from build123d import *

# Parameters (mm, degrees)
ESQUISSE1_R        = 5.74
BOSS_EXTRU_1_DEPTH = 5.5
ESQUISSE2_R        = 11.65
BOSS_EXTRU_2_DEPTH = 8
ESQUISSE3_R        = 8.55
BOSS_EXTRU_3_DEPTH = 35.3
ESQUISSE4_R        = 3.5
BOSS_EXTRU_4_DEPTH = 7.2


with BuildPart() as part:
    # Esquisse1 → Boss.-Extru.1 (new body)
    with BuildSketch(Plane.XY):
        Circle(ESQUISSE1_R)
    extrude(amount=BOSS_EXTRU_1_DEPTH)

    # Esquisse2 → Boss.-Extru.2 (add)
    with BuildSketch(Plane(origin=(0, 0, 0), x_dir=(-1, 0, 0), z_dir=(0, 0, -1))):
        Circle(ESQUISSE2_R)
    extrude(amount=BOSS_EXTRU_2_DEPTH)

    # Esquisse3 → Boss.-Extru.3 (add)
    with BuildSketch(Plane(origin=(0, 0, -8), x_dir=(-1, 0, 0), z_dir=(0, 0, -1))):
        Circle(ESQUISSE3_R)
    extrude(amount=BOSS_EXTRU_3_DEPTH)

    # Esquisse4 → Boss.-Extru.4 (add)
    with BuildSketch(Plane(origin=(0, 0, -43.3), x_dir=(-1, 0, 0), z_dir=(0, 0, -1))):
        with Locations((4.865332224, 0)):
            Circle(ESQUISSE4_R)
    extrude(amount=BOSS_EXTRU_4_DEPTH)


solid = part.part
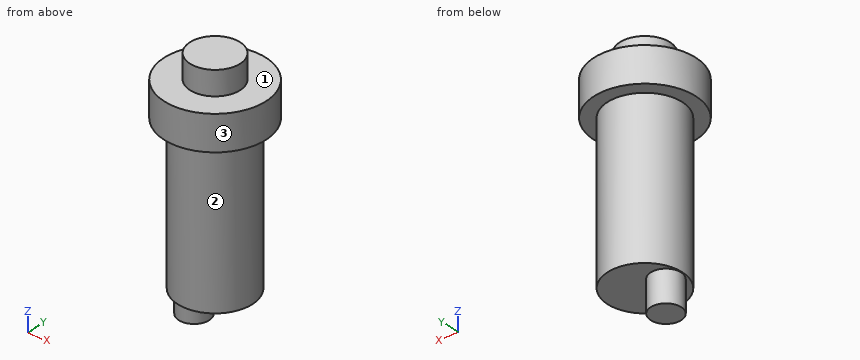
The model under review builds one solid part; all positions refer to its coordinate system, in mm. Face numbers are marked on the shaded views. A direction names the side the tool comes from. Coordinates: 2 decimals unless noted, no trailing zeros. Order: outer loops, then holes, each group sorted by start corner. A loop starts at its lowest first (then second) coordinate and runs counter-clockwise, first axis right, second up. Notation, with made-up numbers: (85.5, -21) -> (137.5, -21) arc R30 ccw to (137.5, 16) -> close; hole circle Ø6 at (-19, 40). An arc over 180 degrees is marked (long way). Answer in a Markdown table with one row per item.
(1) Wall thickness on line 1 along Z through (x, y) = (4.5, 8.25); line 2 along Z through (x, y) = (1.25, 6.75); line 3 along Y through (x, z) = (7.25, -26): over which ranges is each line inside the solid? List them lowest first.
Answers:
| item | result |
|---|---|
| line 1 | -8 to 0 |
| line 2 | -43.3 to 0 |
| line 3 | -4.53 to 4.53 |
(2) Consider section A-A (y = 0). Write out the cut boundary in (x, z).
Answers:
| item | result |
|---|---|
| outline | (-11.65, -8) -> (-8.55, -8) -> (-8.55, -43.3) -> (-8.37, -43.3) -> (-8.37, -50.5) -> (-1.37, -50.5) -> (-1.37, -43.3) -> (8.55, -43.3) -> (8.55, -8) -> (11.65, -8) -> (11.65, 0) -> (5.74, 0) -> (5.74, 5.5) -> (-5.74, 5.5) -> (-5.74, 0) -> (-11.65, 0) -> close |
(3) Machinability: for the marked faces 1, 2 and 3, which of the approach directions +Z, -Z, +X, -X, +Y, -Y give a long, thin tool a straight path to every point of the face, cutting with its end or side? Answer none if there is none.
Answers:
| item | result |
|---|---|
| face 1 | +Z |
| face 2 | -Z |
| face 3 | +Z, -Z |
(4) Consider section B-B (x = 0). Write out the cut boundary in (y, z).
Answers:
| item | result |
|---|---|
| outline | (-11.65, -8) -> (-8.55, -8) -> (-8.55, -43.3) -> (8.55, -43.3) -> (8.55, -8) -> (11.65, -8) -> (11.65, 0) -> (5.74, 0) -> (5.74, 5.5) -> (-5.74, 5.5) -> (-5.74, 0) -> (-11.65, 0) -> close |
(5) Consider section C-C (z = -7). Write out the cut boundary in (x, y).
Answers:
| item | result |
|---|---|
| outline | circle Ø23.3 at (0, 0) |
(6) Consider section D-D (x = 4.5). Write out the cut boundary in (y, z), plus the area to 3 significant figures.
Answers:
| item | result |
|---|---|
| outline | (-10.75, -8) -> (-7.27, -8) -> (-7.27, -43.3) -> (7.27, -43.3) -> (7.27, -8) -> (10.75, -8) -> (10.75, 0) -> (3.56, 0) -> (3.56, 5.5) -> (-3.56, 5.5) -> (-3.56, 0) -> (-10.75, 0) -> close |
| area | 724 mm² |
(7) Insertion check: pin 1 (8 mm diameter, centred on x = 5.5, y = -3.5, fed in from +Z); pin 2 (5 mm diameter, centred on y = -7, z = -27.5, fed in from -X); pin 3 (3 mm diameter, centred on x = 6, y = -2.5, fed in from -Z); pin 4 (2 mm diameter, centred on x = 0.5, y = 8.5, fed in from +Z). Each pin has a flat end and moves straight along its axis. Give the tip position at first contact, or say it passes through.
Answers:
| item | result |
|---|---|
| pin 1 | z = 5.5 |
| pin 2 | x = -7.27 |
| pin 3 | z = -43.3 |
| pin 4 | z = 0 |
